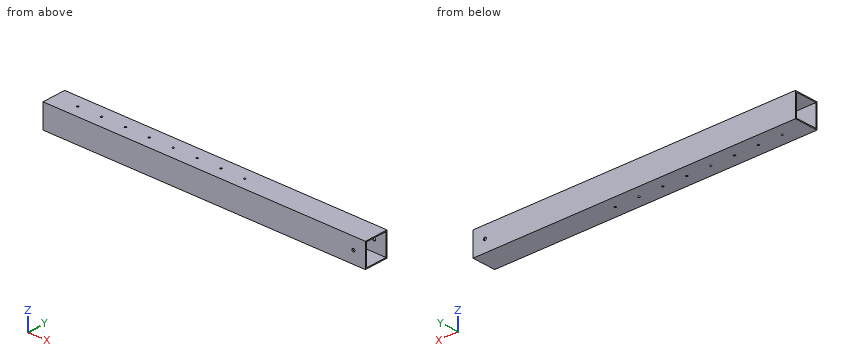
```python
from build123d import *

# Parameters (mm, degrees)
F0_W     = 152.4
F0_H     = 152.4
F0_W_2   = 139.7
F0_H_2   = 139.7
F1_DEPTH = 2057.4
F3_D     = 12.7
F5_D     = 19.05


with BuildPart() as f1:
    # F0 (on Right) → F1 (new body)
    with BuildSketch(Plane.YZ):
        Rectangle(F0_W, F0_H)
        Rectangle(F0_W_2, F0_H_2, mode=Mode.SUBTRACT)
    extrude(amount=F1_DEPTH)

    # F3 (through all)
    with Locations(Plane.XY.offset(76.2)):
        with Locations((152.4, 0), (304.8, 0), (457.2, 0), (609.6, 0), (762, 0), (914.4, 0), (1066.8, 0), (1219.2, 0)):
            Hole(F3_D / 2)

    # F5 (through all)
    with Locations(Plane(origin=(0, 76.2, 0), x_dir=(-1, 0, 0), z_dir=(0, 1, 0))):
        with Locations((-1981.2, 0)):
            Hole(F5_D / 2)


solid = f1.part
```
Geometry: final body of the model. Coordinates: model frame, mm. Round coordinates to 2 decimals unless told otherwise and drop trailing zeros. Write each loop counter-clockwise with the first axis right and the second up, starting at its lowest first coordinate (ties: lowest second). Pieces come first, ordered by that corner, then holes. Notation, with made-up numbers: (62, 64) -> (119, 64) arc R21 cw to (119, 68) -> close; hole circle Ø7 at (87, 46.25). An arc over 180 degrees is marked (long way). Use CSV: the item, a comma, the result in double quotes. Start each with the question number.
Q1. Line query: L1, parallel to Z at x = 280, y = -58.5; L2, parallel to Y at x = 1219, z = 74. Output: solid intervals per line, ascending.
Q2. Section A-A (z = -49.5). Return loops of the section in (x, y).
Q3. Section C-C (x = 267). Return loops of the section in (y, z), plus the area to 3 significant figures.
Result sheet:
1,L1,"-76.2 to -69.85, 69.85 to 76.2"
1,L2,"-76.2 to -6.35, 6.35 to 76.2"
2,outline,"(0, -76.2) -> (2057.4, -76.2) -> (2057.4, -69.85) -> (0, -69.85) -> close; (0, 69.85) -> (2057.4, 69.85) -> (2057.4, 76.2) -> (0, 76.2) -> close"
3,outline,"(-76.2, -76.2) -> (76.2, -76.2) -> (76.2, 76.2) -> (-76.2, 76.2) -> close; hole (-69.85, -69.85) -> (69.85, -69.85) -> (69.85, 69.85) -> (-69.85, 69.85) -> close"
3,area,"3,710 mm²"
